from build123d import *

# Parameters (mm, degrees)
F0_R          = 6.35
F1_DEPTH      = 23.876
F2_R          = 6.35
F2_R_2        = 5.588
F3_DEPTH      = 22.3012
F4_R          = 5.842
F4_R_2        = 4.953
F5_DEPTH      = 0.635
F6_R          = 1.17475
F7_DEPTH      = 5.7404
F7_DEPTH_BACK = 0.0508
F8_R          = 5.715
F8_R_2        = 4.572
F9_DEPTH      = 5.6896
F10_R         = 5.08
F10_R_2       = 4.572
F11_DEPTH     = 4.0894
F12_W         = 7.8048733994
F12_H         = 4.4421355706
F13_DEPTH     = 5.6896
F14_R         = 5.08
F14_R_2       = 4.953
F15_DEPTH     = 1.778
F16_SIZE      = 0.12699
F17_W         = 1.143
F17_H         = 9.652
F18_DEPTH     = 23.877
F19_W         = 1.016
F19_H         = 1.524
F20_DEPTH     = 21.9456
F21_W         = 1.016
F21_H         = 1.5748
F22_DEPTH     = 1.9304
F23_W         = 1.016
F23_H         = 1.778
F24_DEPTH     = 21.336
F25_R         = 0.635
F26_DEPTH     = 21.2852
F29_W         = 1.1630140017
F29_H         = 0.8712620474
F30_DEPTH     = 25.4


# Not quite as in the source:
# - a fillet or chamfer is up to 0.001 mm smaller than in the source, because OpenCascade refuses the exact size


with BuildPart() as f1:
    # F0 (on Top) → F1 (new body)
    with BuildSketch(Plane.XY):
        Circle(F0_R)
    extrude(amount=-F1_DEPTH)

    # F2 (on Top) → F3 (cut)
    with BuildSketch(Plane.XY):
        Circle(F2_R)
        Circle(F2_R_2, mode=Mode.SUBTRACT)
    extrude(amount=-F3_DEPTH, mode=Mode.SUBTRACT)

    # F4 (on face) → F5 (cut)
    with BuildSketch(Plane.XY.offset(-22.3012)):
        Circle(F4_R)
        Circle(F4_R_2, mode=Mode.SUBTRACT)
    extrude(amount=F5_DEPTH, mode=Mode.SUBTRACT)

    # F6 (on Front) → F7 (cut, two sides)
    with BuildSketch(Plane.XZ) as f7_sk:
        with Locations((0, -19.9009)):
            Circle(F6_R)
        with Locations((0, -16.8529)):
            Circle(F6_R)
        with Locations((0, -13.8049)):
            Circle(F6_R)
        with Locations((0, -10.7569)):
            Circle(F6_R)
        with Locations((0, -7.7089)):
            Circle(F6_R)
    extrude(amount=F7_DEPTH, mode=Mode.SUBTRACT)
    extrude(f7_sk.sketch, amount=-F7_DEPTH_BACK, mode=Mode.SUBTRACT)

    # F8 (on face) → F9 (cut, symmetric)
    with BuildSketch(Plane.XY):
        Circle(F8_R)
        Circle(F8_R_2, mode=Mode.SUBTRACT)
    extrude(amount=F9_DEPTH, both=True, mode=Mode.SUBTRACT)

    # F10 (on face) → F11 (join)
    with BuildSketch(Plane.XY):
        Circle(F10_R)
        Circle(F10_R_2, mode=Mode.SUBTRACT)
    extrude(amount=-F11_DEPTH)

    # F12 (on Front) → F13 (cut, symmetric)
    with BuildSketch(Plane.XZ):
        with Locations((-3.1404366997, -0.3189322147)):
            Rectangle(F12_W, F12_H)
    extrude(amount=F13_DEPTH, both=True, mode=Mode.SUBTRACT)

    # F14 (on face) → F15 (cut)
    with BuildSketch(Plane.XY):
        Circle(F14_R)
        Circle(F14_R_2, mode=Mode.SUBTRACT)
    extrude(amount=-F15_DEPTH, mode=Mode.SUBTRACT)

    # F16 (size 0.127 in the source; OpenCascade refuses exactly that, so slightly less here)
    f16_edges = [f1.edges().sort_by_distance(p)[0] for p in [
        (4.953, 0, -1.778),
    ]]
    chamfer(f16_edges, length=F16_SIZE)

    # F17 (on face) → F18 (cut, through all)
    with BuildSketch(Plane(origin=(0, 0, -23.876), x_dir=(1, 0, 0), z_dir=(0, 0, -1))):
        with Locations((0.1905, -1.524)):
            Rectangle(F17_W, F17_H)
    extrude(amount=-F18_DEPTH, mode=Mode.SUBTRACT)

    # F19 (on face) → F20 (cut)
    with BuildSketch(Plane.XY.offset(-2.54)):
        with Locations((-0.889, 4.3036923515)):
            Rectangle(F19_W, F19_H)
    extrude(amount=-F20_DEPTH, mode=Mode.SUBTRACT)

    # F21 (on face) → F22 (cut)
    with BuildSketch(Plane.XZ.offset(-5.0656923515)):
        with Locations((-0.889, -23.0886)):
            Rectangle(F21_W, F21_H)
    extrude(amount=-F22_DEPTH, mode=Mode.SUBTRACT)

    # F23 (on face) → F24 (cut, through all)
    with BuildSketch(Plane.XY.offset(-2.54)):
        with Locations((-0.889, 1.143)):
            Rectangle(F23_W, F23_H)
    extrude(amount=-F24_DEPTH, mode=Mode.SUBTRACT)

    # F25 (on face) → F26 (join)
    with BuildSketch(Plane(origin=(0, 0, -23.876), x_dir=(1, 0, 0), z_dir=(0, 0, -1))):
        with Locations((0.762, -1.27)):
            Circle(F25_R)
    extrude(amount=-F26_DEPTH)

    # F27 (on Right) → F28 (revolve, cut)
    with BuildSketch(Plane.YZ):
        with BuildLine():
            Line((1.4259085423, -23.876), (1.4259085423, -23.368))
            ThreePointArc((1.4259085423, -23.368), (0.2592411198, -23.5154965988), (-0.8600914577, -23.876))
            Line((-0.8600914577, -23.876), (1.4259085423, -23.876))
        make_face()
    revolve(axis=Axis((0, 1.4259085423, -23.622), (0, 0, -1)), mode=Mode.SUBTRACT)

    # F29 (on face) → F30 (cut)
    with BuildSketch(Plane.XY.offset(-5.6896)):
        with Locations((-0.8154929991, 5.274676485)):
            Rectangle(F29_W, F29_H)
    extrude(amount=-F30_DEPTH, mode=Mode.SUBTRACT)


solid = f1.part
Design review of the part built by this model. Coordinates are the model's own, in mm. A direction names the side the tool comes from. Coordinates: 2 decimals unless noted, no trailing zeros. Write each loop counter-clockwise with the first axis right and the second up, starting at its lowest first coordinate (ties: lowest second). Pieces come first, ordered by that corner, then holes. Notation, with made-up numbers: (-33, -35) -> (17, -35) arc R17 cw to (17, -5) -> close; hole circle Ø10 at (-11.75, -22.75). An arc over 180 degrees is marked (long way). Write each question's results on one line, items separated by ' | '. Start each with the question number.
(1) Take a section at A-A on z = -3.5. Write out the cut boundary in (x, y) (3 decimals), and give its area (3 significant figures).
(2) Take a section at C-C on y = -4. Give the number of separate pieces and of enclosed holes in the cut face, and give its area (3 significant figures).
(3) The part is to be moulded in two halves that separate along Z. For faces 1 (the face through (-1.397, 5, -13)), 2 (the face through (2, 0, 0)), 3 (the face through (-1.174, -3.358, -7.657)), 4 (the face through (-4.2, -2.3, -4.089)), say which applies: pulls with the +Z half, pulls with the -Z half, needs draft (parallel to the pull), parting line crosses it, or undercut.
(4) For line 1 along Z through (x, y) = (0, -4.15); line 2 along X through (y, z) = (0, -12); line 3 along X through (y, z) = (-2, -9.75), list the stretches that pass through material, from the lowest coordinate up. Write a range as from..to.
(5) Take a section at B-B on x = -3.5. Write out the cut boundary in (y, z), and give its area (3 significant figures).
(6) Tool access review of faces 5 (the face through (0.2, -3.302, -15.3)), 6 (the face through (2.706, 4.889, -13.566)), 7 (the face through (4.95, -0.1, -0.81)): name each direction out of +Z, -Z, +X, -X, +Y, -Y from which nothing blocks a thin tool from reaching the whole face with its end or side.
(7) Clearance check with flat-ended pins moving along their axes: P1, Ø0.5, axis at x = 1, z = -14, coming from the -Y side; P2, Ø1.3, axis at x = 0, z = -12, coming from the +Y side; P3, Ø3, axis at x = 0, z = -10.76, coming from the +Y side. State where each tip first meets the part, or that it passes through.
Results found:
1) outline: (-1.397, 0.254) -> (-1.397, 2.032) -> (-0.381, 2.032) -> (-0.381, 3.542) -> (-1.397, 3.542) -> (-1.397, 4.884) arc R5.08 ccw (long way) to (0.762, 5.023) -> (0.762, 1.905) arc R0.635 ccw to (0.762, 0.635) -> (0.762, -3.302) -> (-0.381, -3.302) -> (-0.381, 0.254) -> close | area: 68.9 mm2
2) separate pieces: 1 | enclosed holes: 5 | area: 145 mm2
3) face 1: needs draft | face 2: pulls with the +Z half | face 3: undercut | face 4: undercut
4) line 1: z = -23.88..-21.08, -18.73..-18.03, -15.68..-14.98, -12.63..-11.93, -9.58..-8.88, -6.53..-2.54 | line 2: x = -5.59..-0.38, 0.76..5.59 | line 3: x = -5.22..-0.61, 0.76..5.22
5) outline: (-5.3, -23.88) -> (5.3, -23.88) -> (5.3, -22.3) -> (3.5, -22.3) -> (3.5, -21.67) -> (4.36, -21.67) -> (4.36, -5.69) -> (2.94, -5.69) -> (2.94, -4.09) -> (3.68, -4.09) -> (3.68, -2.54) -> (-3.68, -2.54) -> (-3.68, -4.09) -> (-2.94, -4.09) -> (-2.94, -5.69) -> (-4.36, -5.69) -> (-4.36, -21.67) -> (-3.5, -21.67) -> (-3.5, -22.3) -> (-5.3, -22.3) -> close | area: 181 mm2
6) face 5: +Z, -Z | face 6: +Z | face 7: +Z, +X
7) P1: stops at y = -5.48 | P2: stops at y = 3.54 | P3: stops at y = 5.54
